Could you check a few things on this model? Use its own coordinates, in mm. Face numbers are marked on the shaded views. A direction names the side the tool comes from. Give positions to 0.01 mm unless a question says otherwise; leave off trailing zeros. Write each loop counter-clockwise with the first axis right and the second up, starting at its lowest first coordinate (ties: lowest second). Pieces come first, ordered by that corner, then holes. Notation, with made-up numbers: (27, 30.25) - (75, 30.25) arc R28 ccw to (75, 49.25) - close; hole circle Ø3 at (33.5, -35). An arc over 180 degrees is marked (long way). Answer as CSV lines item,"result". Start each with the question number.
Q1. Imagine slicing it at D-D on z = -13.5. List the corners of the cut face in (x, y) for me, and give its area (3 significant figures).
Q2. If I drill on line 1 along X through (y, z) = (25, 3.75); line 2 along Y through (x, z) = (-10, 4.15); line 3 along Y through (x, z) = (10, 0.8), over which ranges is the centre line in solid material (lowest first)?
Q3. Imagine slicing it at C-C on x = 0. List the corners of the cut face in (y, z) for me, and give its area (3 significant figures).
Q4. Imagine slicing it at A-A on y = -25. List the corners of the cut face in (x, z) for me, and give its area (3 significant figures).
Q5. Will these pins go through, and if not, where does the flat tip stop? pin 1 Ø4 at (x, y) = (-25, 10) entering from -Z; pin 2 Ø2.5 at (x, y) = (-10, 25) entering from -Z; pin 3 Ø9 at (x, y) = (25, -10) entering from +Z; pin 4 Ø4 at (x, z) = (16.5, -25) entering from -Y.
Q6. On a 3-axis mill with a long thin cutter (end or side, diameter ignored), from which of +Z, -Z, +X, -X, +Y, -Y can I reach the whole of each face in a straight line? I mean the marked faces 1, 2 and 3. Say none if no direction works.
Q7. Imagine slicing it at B-B on x = -25. List the corners of the cut face in (y, z) for me.
Autodesk Inventor part; units mm, degrees
ref_plane "YZ Plane" through (0, 0, 0) normal (1, 0, 0) x (0, 1, 0)
ref_plane "XZ Plane" through (0, 0, 0) normal (0, 1, 0) x (-1, 0, 0)
ref_plane "XY Plane" through (0, 0, 0) normal (0, 0, 1) x (1, 0, 0)
ref_plane "Work Plane1" through (0, 0, 0) normal (0, 0, 1) x (1, 0, 0)
sketch "Sketch1" plane through (0, 0, 0) normal (0, 0, 1) x (1, 0, 0)
  circle A0 centre (-10, -25) radius 1.45
  circle A1 centre (-10, 25) radius 1.45
  circle A2 centre (10, 25) radius 1.45
  circle A3 centre (10, -25) radius 1.45
  circle A4 centre (-25, 25) radius 2.325
  circle A5 centre (25, -25) radius 2.325
  circle A6 centre (-25, -25) radius 2.325
  circle A7 centre (25, 25) radius 2.325
  line L0 (28, 30) -> (30, 28)
  line L1 (28, 30) -> (-28, 30)
  line L2 (-30, 28) -> (-28, 30)
  line L3 (-30, 28) -> (-30, -28)
  line L4 (-28, -30) -> (-30, -28)
  line L5 (-28, -30) -> (28, -30)
  line L6 (30, -28) -> (28, -30)
  line L7 (30, -28) -> (30, 28)
  circle A8 centre (-17.5, -17.5) radius 1.95
  circle A9 centre (17.5, 17.5) radius 1.95
  circle A10 centre (17.5, -17.5) radius 1.95
  circle A11 centre (-17.5, 17.5) radius 1.95
  circle A12 centre (0, 0) radius 7.5
  circle A13 centre (-25.33, -75.26) radius 6.15
  circle A14 centre (25, -10) radius 1.45
  circle A15 centre (-25, -10) radius 1.45
  circle A16 centre (-25, 10) radius 1.45
  circle A17 centre (25, 10) radius 1.45
  line L8 (-28, -30) -> (-31, -30)
  line L9 (-31, -30) -> (-31, 30)
  line L10 (-31, 30) -> (-28, 30)
  line L11 (-28, 30) -> (-28, -30)
  point P0 (0, 0)
  dimension "d0" = 3
extrude "Extrusion1" add sketch "Sketch1" along normal blind 6 contours A4 | A5 | A6 | A7 | L0 L7 L6 L5 L11 L1 | L11 L4 L3 L2 | L2 L3 L4 L8 L9 L10 | A8 | A9 | A10 | A11
ref_plane "Work Plane3" through (0, 0, 19) normal (0, 0, 1) x (1, 0, 0)
sketch "Sketch7" plane through (0, 0, 6) normal (0, 0, 1) x (1, 0, 0)
  circle A0 centre (10, -25) radius 1.45
  circle A1 centre (-10, -25) radius 1.45
  circle A2 centre (-25, -10) radius 1.45
  circle A3 centre (-25, 10) radius 1.45
  circle A4 centre (-10, 25) radius 1.45
  circle A5 centre (10, 25) radius 1.45
  circle A6 centre (25, 10) radius 1.45
  circle A7 centre (25, -10) radius 1.45
  point P0 (0, 0)
hole "Hole1" at (-25, -10, 6) at (-25, 10, 6) at (-10, 25, 6) at (10, 25, 6) at (25, 10, 6) at (25, -10, 6) at (10, -25, 6) at (-10, -25, 6) direction (0, 0, -1) diameter 3.2 end through all counterbore diameter 8 counterbore depth 4
sketch "Sketch10" plane through (-31, -30, 0) normal (-1, 0, 0) x (0, 0, 1)
  line L0 (2, 16) -> (2, 24)
  line L1 (0, 0) -> (0, 60)
  line L2 (0, 0) -> (6, 0)
  line L3 (6, 60) -> (6, 0)
  line L4 (0, 60) -> (6, 60)
  line L5 (6, 0) -> (6, -20)
  line L6 (6, -20) -> (-30, -20)
  line L7 (-30, -20) -> (-30, -83.2379)
  line L8 (-30, -83.2379) -> (-36, -83.2379)
  line L9 (-36, -83.2379) -> (-36, -14)
  line L10 (-36, -14) -> (0, -14)
  line L11 (0, -14) -> (0, 0)
  line L12 (6, 60) -> (6, 0)
  line L13 (0, 0) -> (6, 0)
  point P0 (0, 30)
  dimension "d55" = 20
  dimension "d56" = 90
  dimension "d57" = 6
  dimension "d58" = 90
  dimension "d59" = 90
  dimension "d60" = 90
  dimension "d61" = 30
  dimension "d71" = 6
extrude "Extrusion9" add sketch "Sketch10" against normal up to surface (59 mm away) contours L2 L5 L6 L7 L8 L9 L10 L11
sketch "Sketch11" plane through (-31, -113.2379, -30) normal (0, 0, 1) x (1, 0, 0)
  line L0 (59, 63.2379) -> (59, 0)
  line L1 (0, 63.2379) -> (59, 63.2379)
  line L2 (0, 0) -> (0, 63.2379)
  line L3 (0, 0) -> (59, 0)
  circle A0 centre (31, 31.6189) radius 10
  point P0 (31, 113.2379)
  dimension "d65" = 20
extrude "Extrusion10" cut sketch "Sketch11" against normal blind 10 contours A0
chamfer "Chamfer3" distance 5 angle 45 2 edges at (-1.5, -50, -30) (-1.5, -44, 0)
sketch "Sketch12" plane through (-31, -113.2379, -30) normal (0, 0, 1) x (1, 0, 0)
  line L0 (0, 58.2379) -> (59, 58.2379)
  line L1 (0, 0) -> (0, 58.2379)
  line L2 (0, 0) -> (59, 0)
  line L3 (59, 58.2379) -> (59, 0)
  circle A0 centre (31, 31.6189) radius 10
  line L4 (51, 51.6189) -> (11, 51.6189)
  line L5 (11, 51.6189) -> (11, 11.6189)
  line L6 (11, 11.6189) -> (51, 11.6189)
  line L7 (51, 11.6189) -> (51, 51.6189)
  line L8 (51, 51.6189) -> (11, 11.6189) construction
  line L9 (11, 51.6189) -> (51, 11.6189) construction
  point P0 (31, 113.2379)
  dimension "d72" = 40
  dimension "d73" = 40
hole "Hole2" at (-20, -101.6189, -30) at (-20, -61.6189, -30) at (20, -61.6189, -30) at (20, -101.6189, -30) direction (0, 0, -1) diameter 4.9 end through all
sketch "Sketch13" plane through (-31, -113.2379, -30) normal (0, 0, 1) x (1, 0, 0)
  circle A0 centre (51, 51.6189) radius 2.45
  circle A1 centre (11, 11.6189) radius 2.45
  circle A2 centre (11, 51.6189) radius 2.45
  circle A3 centre (51, 11.6189) radius 2.45
  line L0 (0, 58.2379) -> (59, 58.2379)
  line L1 (0, 0) -> (0, 58.2379)
  line L2 (0, 0) -> (59, 0)
  line L3 (59, 58.2379) -> (59, 0)
  circle A4 centre (31, 31.6189) radius 10
  circle A5 centre (31, 31.6189) radius 17.5
  line L4 (0, 58.2379) -> (15.0116, 24.5041)
  line L5 (0, 58.2379) -> (59, 58.2379)
  line L6 (59, 58.2379) -> (47.4948, 25.7733)
  point P0 (31, 113.2379)
  dimension "d81" = 35
extrude "Extrusion11" cut sketch "Sketch13" against normal through all contours L4 A5 L6 L3 L2 L1
equation "\"d57\" = d1"
equation "\"d71\" = d1"
properties part number "cellSTORM_UC2_Sample_arm_ptycho"
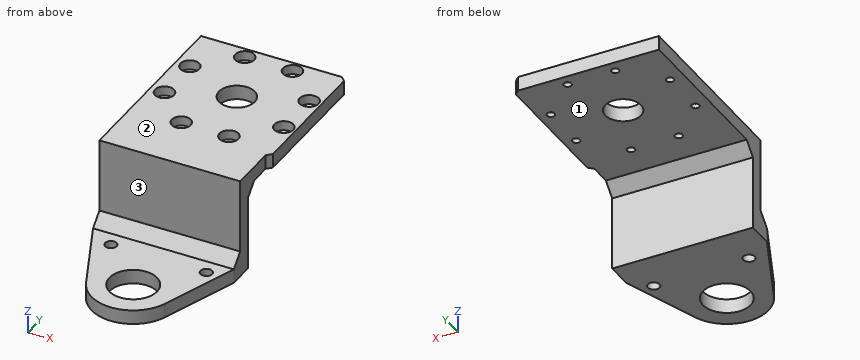
Conclusion:
1,outline,"(-31, -50) - (28, -50) - (28, -44) - (-31, -44) - close"
1,area,"354 mm^2"
2,line 1,"-31 to -14, -6 to 6, 14 to 30"
2,line 2,"-50 to -29, -21 to 21, 29 to 30"
2,line 3,"-50 to -26.6, -23.4 to 23.4, 26.6 to 30"
3,outline,"(-99.12, -36) - (-91.62, -36) - (-91.62, -30) - (-99.12, -30) - close; (-71.62, -36) - (-44, -36) - (-44, -5) - (-39, 0) - (-7.5, 0) - (-7.5, 6) - (-50, 6) - (-50, -25) - (-55, -30) - (-71.62, -30) - close; (7.5, 0) - (30, 0) - (30, 6) - (7.5, 6) - close"
3,area,"806 mm^2"
4,outline,"(-31, 0) - (-11.6, 0) - (-11.6, 2) - (-14, 2) - (-14, 6) - (-31, 6) - close; (-8.4, 0) - (8.4, 0) - (8.4, 2) - (6, 2) - (6, 6) - (-6, 6) - (-6, 2) - (-8.4, 2) - close; (11.6, 0) - (30, 0) - (30, 6) - (14, 6) - (14, 2) - (11.6, 2) - close"
4,area,"289 mm^2"
5,pin 1,"z = 0"
5,pin 2,"through"
5,pin 3,"z = 6"
5,pin 4,"y = -52"
6,face 1,"-Z, +X, -X, +Y"
6,face 2,"+Z, +X, -X, +Y, -Y"
6,face 3,"+Z, +X, -X, -Y"
7,outline,"(-68.48, -36) - (-44, -36) - (-44, -5) - (-39, 0) - (-11.6, 0) - (-11.6, 2) - (-14, 2) - (-14, 6) - (-50, 6) - (-50, -25) - (-55, -30) - (-68.48, -30) - close; (-8.4, 0) - (8.4, 0) - (8.4, 2) - (6, 2) - (6, 6) - (-6, 6) - (-6, 2) - (-8.4, 2) - close; (11.6, 0) - (30, 0) - (30, 6) - (14, 6) - (14, 2) - (11.6, 2) - close"
